For this review, use the dimensioned drawing (mm, ordinates from the lowest corner) and the shaded views. A direction names the side the tool comes from. Coordinates: 2 decimals unless noted, no trailing zeros. Order: outer loops, then holes, each group sorted by start corner. A loop starts at its lowest first (then second) coordinate and runs counter-clockwise, first axis right, second up. Notation, with made-up numbers: M -37,-19.5 L 0,-19.5 A28 ccw 0,12.5 Z; hole C 50,12.25 d1. An arc over 180 degrees is marked long. One line per item, written item: value.
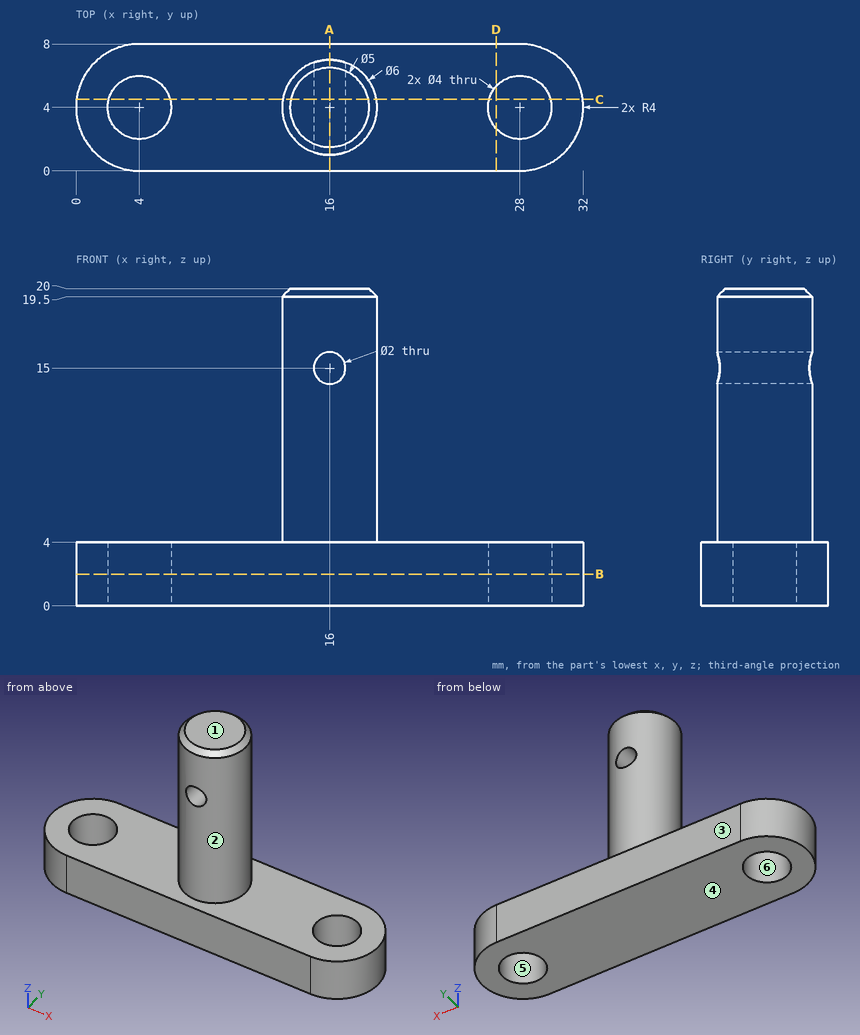
(1) Tool access review of the marked faces 1 and 2: name each direction out of +Z, -Z, +X, -X, +Y, -Y from which nothing blocks a thin tool from reaching the whole face with its end or side.
Geometry results:
face 1: +Z, +X, -X, +Y, -Y
face 2: +Z
(2) We need section A-A, the plane x = 16. State the section outline as (y, z) points.
Geometry results:
outline: M 0,0 L 8,0 L 8,4 L 7,4 L 7,14 L 1,14 L 1,4 L 0,4 Z; M 1,16 L 7,16 L 7,19.5 L 6.5,20 L 1.5,20 L 1,19.5 Z
(3) For L1, parallel to X at y = 4, z = 3.1; L2, parallel to Y at x = 4, z = 3.05; L3, parallel to Z at x = 21, y = 7.25, list the stretches that pass through material, from the lowest coordinate up.
Geometry results:
L1: x = 0 to 2, 6 to 26, 30 to 32
L2: y = 0 to 2, 6 to 8
L3: z = 0 to 4
(4) Insertion check: pin 1 Ø4 at (x, y) = (10, 6.5) entering from +Z; pin 2 Ø2 at (y, z) = (5.5, 15.5) entering from -X; pin 3 Ø2 at (y, z) = (1.5, 9.5) entering from +X. Each pin has a flat end and moves straight along its axis. Give the tip position at first contact, or say it passes through.
Geometry results:
pin 1: stops at z = 4
pin 2: stops at x = 13.04
pin 3: stops at x = 18.6
(5) We need section C-C, the plane y = 4.5. Count the separate pieces of the cut face and the enclosed holes in it, plus the area to 3 significant figures.
Geometry results:
separate pieces: 3
enclosed holes: 1
area: 188 mm2
(6) Mouldability with a two-part tool opening along Y and no side actions: class the marked faces 3, 4, 5 and 6 as +Y half, -Y half, draft (parallel to the pull), parting line (faces both ways), or undercut.
Geometry results:
face 3: +Y half
face 4: draft
face 5: undercut
face 6: undercut
(7) We need section B-B, the plane z = 2. State the section outline as (x, y) points.
Geometry results:
outline: M 4,0 L 28,0 A4 ccw 28,8 L 4,8 A4 ccw Z; hole C 4,4 d4; hole C 28,4 d4
(8) We need section D-D, the plane x = 26.5. State the section outline as (y, z) points, plus the area to 3 significant figures.
Geometry results:
outline: M 0,0 L 2.68,0 L 2.68,4 L 0,4 Z; M 5.32,0 L 8,0 L 8,4 L 5.32,4 Z
area: 21.4 mm2
